Autodesk Inventor part; units mm, degrees
ref_plane "YZ Plane" through (0, 0, 0) normal (1, 0, 0) x (0, 1, 0)
ref_plane "XZ Plane" through (0, 0, 0) normal (0, 1, 0) x (-1, 0, 0)
ref_plane "XY Plane" through (0, 0, 0) normal (0, 0, 1) x (1, 0, 0)
sketch "Sketch1" plane through (0, 0, 0) normal (0, 1, 0) x (-1, 0, 0)
  line L0 (-26, 44) -> (26, 44)
  line L1 (29, 41) -> (29, -42)
  line L2 (27, -44) -> (-26, -44)
  line L3 (-29, -41) -> (-29, 41)
  line L4 (-29, 44) -> (29, -44) construction
  line L5 (29, 44) -> (-29, -44) construction
  arc A0 (27, -44) -> (29, -42) centre (27, -42) ccw
  arc A1 (-29, -41) -> (-26, -44) centre (-26, -41) ccw
  arc A2 (-26, 44) -> (-29, 41) centre (-26, 41) ccw
  arc A3 (29, 41) -> (26, 44) centre (26, 41) ccw
  line L6 (31, -42) -> (31, 41)
  arc A4 (31, 41) -> (26, 46) centre (26, 41) ccw
  line L7 (26, 46) -> (-26, 46)
  arc A5 (-26, 46) -> (-31, 41) centre (-26, 41) ccw
  line L8 (-31, 41) -> (-31, -41)
  arc A6 (-31, -41) -> (-26, -46) centre (-26, -41) ccw
  line L9 (-26, -46) -> (27, -46)
  arc A7 (27, -46) -> (31, -42) centre (27, -42) ccw
  point P0 (0, 0)
  dimension "d0" = 58
  dimension "d1" = 88
  dimension "d2" = 2
  dimension "d3" = 3
  dimension "d4" = 2
extrude "Extrusion1" add sketch "Sketch1" along normal blind 1
sketch "Sketch2" plane through (0, 0, 0) normal (0, -1, 0) x (1, 0, 0)
  arc A0 (-26, 46) -> (-31, 41) centre (-26, 41) ccw
  line L0 (-26, 46) -> (26, 46)
  arc A1 (31, 41) -> (26, 46) centre (26, 41) ccw
  line L1 (31, 41) -> (31, -41)
  arc A2 (26, -46) -> (31, -41) centre (26, -41) ccw
  line L2 (26, -46) -> (-27, -46)
  arc A3 (-31, -42) -> (-27, -46) centre (-27, -42) ccw
  line L3 (-31, -42) -> (-31, 41)
  line L4 (-27, -46) -> (26, -46)
  line L5 (31, -41) -> (31, 41)
  line L6 (26, 46) -> (-26, 46)
  line L7 (-31, 41) -> (-31, -42)
  line L8 (-30, -44.5) -> (30, 44.5) construction
  line L9 (30, -44.5) -> (-30, 44.5) construction
  arc A4 (-26, 46) -> (-31, 41) centre (-26, 41) ccw
  arc A5 (31, 41) -> (26, 46) centre (26, 41) ccw
  arc A6 (26, -44) -> (29, -41) centre (26, -41) ccw
  arc A7 (26, -46) -> (31, -41) centre (26, -41) ccw
  arc A8 (-31, -42) -> (-27, -46) centre (-27, -42) ccw
  line L10 (26, 42) -> (-26, 42)
  arc A9 (-26, 42) -> (-27, 41) centre (-26, 41) ccw
  line L11 (-27, 41) -> (-27, -42)
  line L12 (-27, -42) -> (26, -42)
  arc A10 (26, -42) -> (27, -41) centre (26, -41) ccw
  line L13 (27, -41) -> (27, 41)
  arc A11 (27, 41) -> (26, 42) centre (26, 41) ccw
  point P0 (0, 0)
  dimension "d12" = 4
extrude "Extrusion2" add sketch "Sketch2" along normal blind 2.5
sketch "Sketch3" plane through (26, 1, -46) normal (0, 0, -1) x (-1, 0, 0)
  line L0 (53, -3.5) -> (53, 0)
  line L1 (53, 0) -> (0, 0)
  line L2 (0, 0) -> (0, 1.5)
  line L3 (0, 1.5) -> (53, 1.5)
  line L4 (53, 1.5) -> (53, 0)
  point P0 (26, -1)
  dimension "d9" = 1.5
extrude "Extrusion3" add sketch "Sketch3" against normal blind 2
sketch "Sketch4" plane through (0, -2.5, 0) normal (0, -1, 0) x (1, 0, 0)
  line L0 (26, 46) -> (-26, 46)
  line L1 (-31, 41) -> (-31, -42)
  line L2 (-27, -46) -> (26, -46)
  line L3 (31, -41) -> (31, 41)
  line L4 (30, 44.5) -> (-30, -44.5) construction
  line L5 (-30, 44.5) -> (30, -44.5) construction
  line L6 (-27, -46) -> (26, -46)
  line L7 (-31, 41) -> (-31, -42)
  arc A0 (26, -46) -> (31, -41) centre (26, -41) ccw
  arc A1 (-31, -42) -> (-27, -46) centre (-27, -42) ccw
  arc A2 (-26, 46) -> (-31, 41) centre (-26, 41) ccw
  arc A3 (31, 41) -> (26, 46) centre (26, 41) ccw
  arc A4 (26, -46) -> (31, -41) centre (26, -41) ccw
  line L8 (26, -42) -> (-27, -42)
  arc A5 (-31, -42) -> (-27, -46) centre (-27, -42) ccw
  arc A6 (-26, 46) -> (-31, 41) centre (-26, 41) ccw
  arc A7 (31, 41) -> (26, 46) centre (26, 41) ccw
  line L9 (26, 46) -> (-26, 46)
  point P0 (0, 0)
  point P1 (-31, 41)
  point P2 (-31, -42)
  point P3 (26, -46)
extrude "Extrusion4" add sketch "Sketch4" along normal blind 2.5
sketch "Sketch5" plane through (26, 2.5, -46) normal (0, 0, -1) x (-1, 0, 0)
  line L0 (53, -7.5) -> (0, -7.5)
  line L1 (19, -7.5) -> (33, -7.5)
  line L2 (33, -7.5) -> (33, -4)
  line L3 (33, -4) -> (19, -4)
  line L4 (19, -4) -> (19, -7.5)
  line L5 (19, -7.5) -> (33, -4) construction
  line L6 (33, -7.5) -> (19, -4) construction
  point P0 (26, -2.5)
  point P1 (26, -5.75)
  dimension "d16" = 14
  dimension "d17" = 0
  dimension "d18" = 3.5
extrude "Extrusion5" cut sketch "Sketch5" against normal blind 10
properties part number "piholder-proto-v3"
Work out the finished part from the listing and answer in its coordinate system (mm). A direction names the side the tool comes from. Coordinates: 2 decimals unless noted, no trailing zeros. Order: outer loops, then holes, each group sorted by start corner. A loop starts at its lowest first (then second) coordinate and runs counter-clockwise, first axis right, second up. Notation, with made-up numbers: M -3,82.5 L 38,82.5 A11 ccw 38,93.5 Z; hole C -28.5,35.25 d7. An arc over 180 degrees is marked long. Use CSV: the item, a comma, the result in double quotes.
1) Flat-ended cylindrical pins translate along their axes: pin 1 Ø1.2 at (x, z) = (2, -44) entering from -Y; pin 2 Ø1.6 at (y, z) = (2, -45.5) entering from +X; pin 3 Ø1.6 at (y, z) = (2, -45.5) entering from -X. Find the tip coordinate at first contact, or state that the pin passes through.
Worked out:
pin 1,"stops at y = -1.5"
pin 2,"stops at x = 26"
pin 3,"stops at x = -27"
2) For faces 1 (the face through (-1, -1, -42)), 2 (the face through (-1, -1, -46)), 3 (the face through (-7, -4, -41)), determine the directions among +Z, -Z, +X, -X, +Y, -Y from which every point of the face is accessible in a straight line to the end or side of a thin tool.
Worked out:
face 1,"+Y"
face 2,"-Z, +X, -X, +Y, -Y"
face 3,"-Z, -Y"
3) Consider line 1 (X direction, y = -1.5, z = -19); line 2 (Z direction, x = -14.5, y = -0.75); line 3 (X direction, y = 0.25, z = 33). Determine where each line is inside the solid, lowest interval first. Write a range as [from, to].
Worked out:
line 1,"x = [-31, -27], [27, 31]"
line 2,"z = [-46, -42], [42, 46]"
line 3,"x = [-31, -29], [29, 31]"
4) Section A-A on z = -40 is taken. Write down the section's boundary in (x, y), plus the area to 3 significant figures.
Worked out:
outline,"M -31,-5 L -7,-5 L -7,-2.5 L -27,-2.5 L -27,0 L -29,0 L -29,1 L -31,1 Z; M 7,-5 L 31,-5 L 31,1 L 29,1 L 29,0 L 27,0 L 27,-2.5 L 7,-2.5 Z"
area,"144 mm^2"
5) Section C-C on y = -4 is taken. Write down the section's boundary in (x, z), plus the area to 3 significant figures.
Worked out:
outline,"M -31,-42 A4 ccw -27,-46 L -7,-46 L -7,-36 L 7,-36 L 7,-46 L 26,-46 A5 ccw 31,-41 L 31,41 A5 ccw 26,46 L -26,46 A5 ccw -31,41 Z"
area,"5,540 mm^2"
6) Section B-B on x = 19 is taken. Write down the section's boundary in (y, z), plus the area to 3 significant figures.
Worked out:
outline,"M -5,-46 L 2.5,-46 L 2.5,-44 L 0,-44 L 0,-42 L -2.5,-42 L -2.5,42 L 0,42 L 0,44 L 1,44 L 1,46 L -5,46 Z"
area,"257 mm^2"
7) Determine the mould class of faces 4 (the face through (-28.1, 0.49, 43.14)), 5 (the face through (0, -2, 46)), 6 (the face through (7, -4, -41)) for opening direction Z: released by +Z, released by -Z, zero draft, split by the parting line, or undercut.
Worked out:
face 4,"undercut"
face 5,"released by +Z"
face 6,"zero draft"
